```python
from build123d import *

# Parameters (mm, degrees)
REVOLVE_THIN2_START         = 6.945845758
REVOLVE_THIN2_OUTLINE_R     = 25
REVOLVE_THIN2_OUTLINE_R_2   = 15
REVOLVE_THIN2_DEPTH         = 45
REVOLVE_THIN2_START_2       = 31.945845758
REVOLVE_THIN2_2_OUTLINE_R   = 45
REVOLVE_THIN2_2_OUTLINE_R_2 = 25
REVOLVE_THIN2_2_DEPTH       = 10
FILLET4_R                   = 5


# Read off the part's stored shape, not the designer's step: Revolve-Thin2
with BuildPart() as part:
    # Revolve-Thin2 outline → Revolve-Thin2 (new body)
    with BuildSketch(Plane(origin=(0, 0, 0), x_dir=(1, 0, 0), z_dir=(0, 1, 0)).offset(REVOLVE_THIN2_START)):
        Circle(REVOLVE_THIN2_OUTLINE_R)
        Circle(REVOLVE_THIN2_OUTLINE_R_2, mode=Mode.SUBTRACT)
    extrude(amount=REVOLVE_THIN2_DEPTH)

    # Revolve-Thin2 2 outline → Revolve-Thin2 2 (add)
    with BuildSketch(Plane(origin=(0, 0, 0), x_dir=(1, 0, 0), z_dir=(0, 1, 0)).offset(REVOLVE_THIN2_START_2)):
        Circle(REVOLVE_THIN2_2_OUTLINE_R)
        Circle(REVOLVE_THIN2_2_OUTLINE_R_2, mode=Mode.SUBTRACT)
    extrude(amount=REVOLVE_THIN2_2_DEPTH)

    # Fillet4
    fillet4_edges = [part.edges().sort_by_distance(p)[0] for p in [
        (-45, 41.945845758, 0),
        (-45, 31.945845758, 0),
    ]]
    fillet(fillet4_edges, radius=FILLET4_R - 0.0001)  # a hair under: the kernel refuses the full size


solid = part.part
```
Verification items for the finished model (mm, model axes). A direction names the side the tool comes from. Coordinates: 2 decimals unless noted, no trailing zeros. Write each loop counter-clockwise with the first axis right and the second up, starting at its lowest first coordinate (ties: lowest second). Pieces come first, ordered by that corner, then holes. Notation, with made-up numbers: M 27.5,-18 L 40.5,-18 A5 cw 40.5,-10 Z; hole C 49,30 d3. An arc over 180 degrees is marked long. Answer as a JSON object with one key per item and string values. Group by question number.
(1) Material ranges on line 1 (X direction, y = 29.5, z = 0); line 2 (Z direction, x = 0, y = 36.5), recorded low to high.
(2) Release check for a two-part mould opening along Z. For faces 1 (the face through (-14.985, 29.131, -0.66)), 2 (the face through (17.22, 31.946, -18.34)), 3 (the face through (23.846, 46.876, -7.509)) record: +Z half, -Z half, draft (parallel to the pull), parting line (faces both ways), or undercut.
(3) Gauge pin test, flat ends, axial feed: pin 1 (6 mm diameter, centred on x = 22, y = 33.5, fed in from -Z); pin 2 (10 mm diameter, centred on y = 29.5, z = -8, fed in from +X); pin 3 (8 mm diameter, centred on y = 47, z = -24.5, fed in from -X). Record the tip position at first contact, or that the pin passes through.
(4) Tool access check on faces 4 (the face through (17.22, 41.946, -18.34)), 5 (the face through (11, 6.946, 11)), 6 (the face through (23.846, 19.271, -7.509)). Record the directions out of +Z, -Z, +X, -X, +Y, -Y that give a thin tool (end or side, any length) a straight path to the whole face; none if there is none.
(5) Cross-section at C-C, the plane y = 25. Record the cut outline in (x, z).
Reply:
{
 "1": {"line 1": "-25 to -15, 15 to 25", "line 2": "-44.98 to -15, 15 to 44.98"},
 "2": {"face 1": "undercut", "face 2": "draft", "face 3": "parting line"},
 "3": {"pin 1": "z = -40.2", "pin 2": "x = 43.75", "pin 3": "x = -14.31"},
 "4": {"face 4": "+Y", "face 5": "+Z, -Z, +X, -X, -Y", "face 6": "-Y"},
 "5": {"outline": "C 0,0 d50; hole C 0,0 d30"}
}
